```python
from build123d import *

# Parameters (mm, degrees)
BOSS_EXTRUDE1_DEPTH = 34
BOSS_EXTRUDE2_DEPTH = 19
SKETCH3_W           = 18
SKETCH3_H           = 8
CUT_EXTRUDE1_DEPTH  = 62.329030646


with BuildPart() as part:
    # Sketch1 → Boss-Extrude1 (new body)
    with BuildSketch(Plane.XY):
        Polygon((-12.5, 20.5), (-12.5, -20.5), (-2.5, -20.5), (12.5, -6.5), (12.5, 20.5), align=None)
    extrude(amount=-BOSS_EXTRUDE1_DEPTH)

    # Sketch2 → Boss-Extrude2 (add)
    with BuildSketch(Plane.ZY.offset(12.5)):
        Polygon((-30, 20.5), (-30, 33.5), (-23, 33.5), (-23, 44.5), (-11, 44.5), (-11, 33.5), (-4, 33.5), (-4, 20.5), align=None)
    extrude(amount=-BOSS_EXTRUDE2_DEPTH)

    # Sketch3 → Cut-Extrude1 (cut, through all)
    with BuildSketch(Plane.ZY.offset(12.5)):
        with Locations((-17, -16.5)):
            Rectangle(SKETCH3_W, SKETCH3_H)
    extrude(amount=-CUT_EXTRUDE1_DEPTH, mode=Mode.SUBTRACT)


solid = part.part
```
For this review, take the finished solid that the model builds, in its own axes (mm). A direction names the side the tool comes from. Coordinates: 2 decimals unless noted, no trailing zeros. Loops run counter-clockwise (first coordinate to the right, second up) from the corner with the lowest first, then second, coordinate; pieces in that order, holes last.
1. Add section A-A, the plane x = -1.75. Give the boundary of the cut face in (y, z), then the cut area to 3 significant figures.
2. Add section D-D, the plane z = -9. Give the boundary of the cut face in (x, y).
3. Add section C-C, the plane y = -15. Give the boundary of the cut face in (x, z), then the cut area to 3 significant figures.
4. Mouldability with a two-part tool opening along Z and no side actions: class faces 1 (the flat face through (-3, 33.5, -8)), 2 (the flat face through (-5, -17, -8)), 3 (the flat face through (-3, -12.5, -17)), 4 (the flat face through (-3, 39, -11)) as +Z half, -Z half, draft (parallel to the pull), parting line (faces both ways), or undercut.
5. Add section B-B, the plane z = -20. Give the boundary of the cut face in (x, y), then the cut area to 3 significant figures.
6. Insertion check: P1, Ø3.5, axis at x = -5.5, z = -25.5, coming from the +Y side; P2, Ø1, axis at y = 26, z = -25.5, coming from the +X side; P3, Ø4, axis at x = -6, y = 29.5, coming from the +Z side. Each pin has a flat end and moves straight along its axis. Give the tip position at first contact, or say it passes through.
7. For faces 5 (the flat face through (-3, 27, -30)), 6 (the flat face through (-12.5, 12, -17)), 7 (the flat face through (-3, 27, -4)), 8 (the flat face through (-5, -17, -26)), 9 (the flat face through (12.5, 7, -17)), list the 3-axis set-ups (+Z, -Z, +X, -X, +Y, -Y) from which the entire face can be reached by the end or side of a thin tool; tool diameter is ignored.
8. For line 1 (Z direction, x = 0.75, y = 29); line 2 (X direction, y = 26, z = -23); line 3 (Y direction, x = -4, z = -25.5), list the stretches that pass through material, from the lowest coordinate up.
Result:
1. outline: (-19.8, -34) - (20.5, -34) - (20.5, -30) - (33.5, -30) - (33.5, -23) - (44.5, -23) - (44.5, -11) - (33.5, -11) - (33.5, -4) - (20.5, -4) - (20.5, 0) - (-19.8, 0) - (-19.8, -8) - (-12.5, -8) - (-12.5, -26) - (-19.8, -26) - close
1. area: 1,710 mm2
2. outline: (-12.5, -12.5) - (6.07, -12.5) - (12.5, -6.5) - (12.5, 20.5) - (6.5, 20.5) - (6.5, 33.5) - (-12.5, 33.5) - close
3. outline: (-12.5, -34) - (3.39, -34) - (3.39, -26) - (-12.5, -26) - close; (-12.5, -8) - (3.39, -8) - (3.39, 0) - (-12.5, 0) - close
3. area: 254 mm2
4. face 1: draft
4. face 2: undercut
4. face 3: undercut
4. face 4: +Z half
5. outline: (-12.5, -12.5) - (6.07, -12.5) - (12.5, -6.5) - (12.5, 20.5) - (6.5, 20.5) - (6.5, 44.5) - (-12.5, 44.5) - close
5. area: 1,260 mm2
6. P1: stops at y = 33.5
6. P2: stops at x = 6.5
6. P3: stops at z = -4
7. face 5: -Z, +X, -X, +Y
7. face 6: +Z, -Z, -X, +Y, -Y
7. face 7: +Z, +X, -X, +Y
7. face 8: +X, -X, -Y
7. face 9: +Z, -Z, +X, +Y, -Y
8. line 1: z = -30 to -4
8. line 2: x = -12.5 to 6.5
8. line 3: y = -12.5 to 33.5
